Here's the drawing with two shaded views (mm, measured from the low corner). I have some questions. A direction names the side the tool comes from. Give positions to 0.01 mm unless a question says otherwise; leave off trailing zeros. Write each loop counter-clockwise with the first axis right and the second up, starting at its lowest first coordinate (ties: lowest second). Pieces come first, ordered by that corner, then holes.
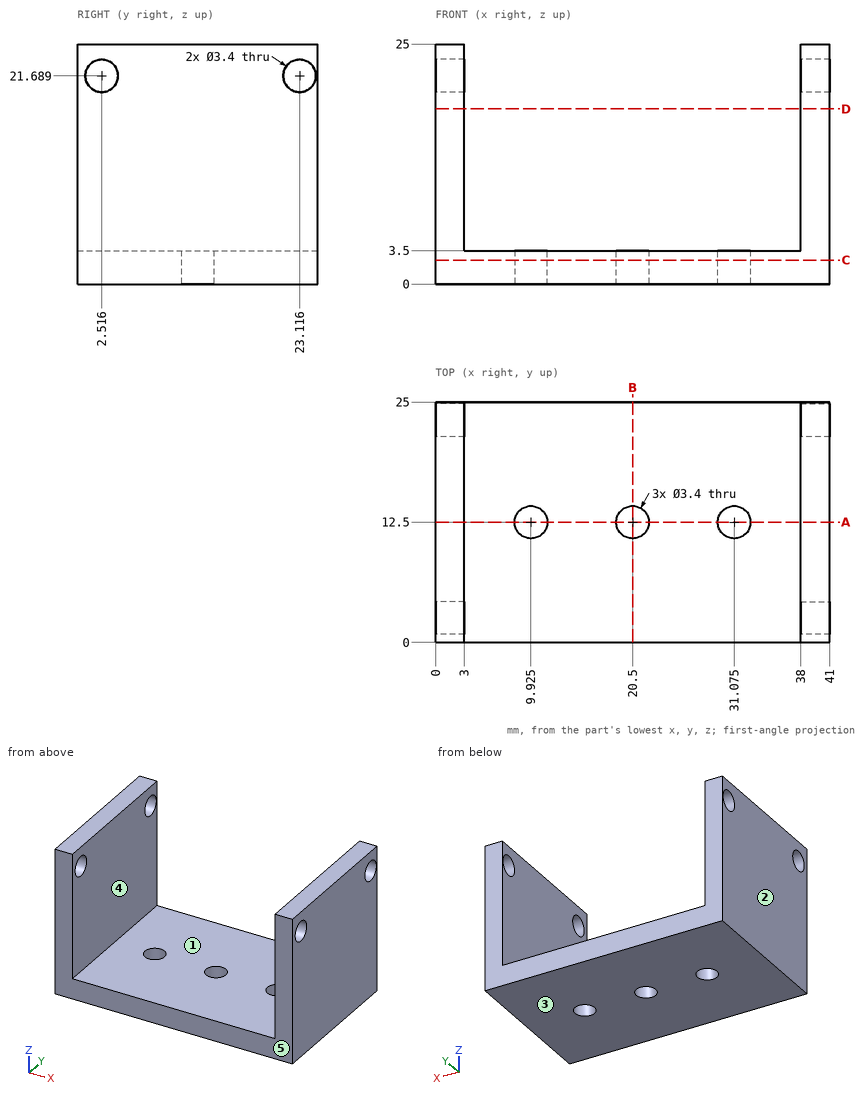
(1) For the marked faces 4 and 5, which set-ups out of +Z, -Z, +X, -X, +Y, -Y let a thin tool reach every point of the face, with its end or its side?
Returned:
face 4: +Z, +Y, -Y
face 5: +Z, -Z, +X, -X, -Y
(2) Imagine slicing it at D-D, the plane z = 18.25. Write out the boundary of the cut face in (x, y).
Returned:
outline: (0, 0) - (3, 0) - (3, 25) - (0, 25) - close; (38, 0) - (41, 0) - (41, 25) - (38, 25) - close
(3) Will these pins go through, and if not, where does the flat tip stop? P1, Ø10, axis at x = 30, z = 13, coming from the +Y side; P2, Ø12.5, axis at x = 23.5, y = 11, coming from the +Z side.
Returned:
P1: passes through
P2: stops at z = 3.5
(4) Imagine slicing it at A-A, the plane y = 12.5. Write out the boundary of the cut face in (x, z) (1 decimal).
Returned:
outline: (0, 0) - (8.2, 0) - (8.2, 3.5) - (3, 3.5) - (3, 25) - (0, 25) - close; (11.6, 0) - (18.8, 0) - (18.8, 3.5) - (11.6, 3.5) - close; (22.2, 0) - (29.4, 0) - (29.4, 3.5) - (22.2, 3.5) - close; (32.8, 0) - (41, 0) - (41, 25) - (38, 25) - (38, 3.5) - (32.8, 3.5) - close
(5) Imagine slicing it at C-C, the plane z = 2.5. Write out the boundary of the cut face in (x, y) (1 decimal), plus the area to 3 significant figures.
Returned:
outline: (0, 0) - (41, 0) - (41, 25) - (0, 25) - close; hole circle Ø3.4 at (9.9, 12.5); hole circle Ø3.4 at (20.5, 12.5); hole circle Ø3.4 at (31.1, 12.5)
area: 998 mm2
(6) Imagine slicing it at B-B, the plane x = 20.5. Write out the boundary of the cut face in (y, z).
Returned:
outline: (0, 0) - (10.8, 0) - (10.8, 3.5) - (0, 3.5) - close; (14.2, 0) - (25, 0) - (25, 3.5) - (14.2, 3.5) - close
(7) If we mould it in two halves opening along X, with no side actions, what happens to the marked faces 1, 2 and 3? For each: +X half, -X half, draft (parallel to the pull), parting line (faces both ways), or undercut.
Returned:
face 1: undercut
face 2: -X half
face 3: draft
(8) If I drill on L1, parallel to X at y = 10, z = 15; L2, parallel to Y at x = 39.5, z = 22 (1 decimal); L3, parallel to Z at x = 14, y = 9.5, over which ranges is the centre line in solid material (lowest first)?
Returned:
L1: x = 0 to 3, 38 to 41
L2: y = 0 to 0.8, 4.2 to 21.4, 24.8 to 25
L3: z = 0 to 3.5
